The drawing under review shows one solid part. Ordinate dimensions are in mm from its lowest x, y, z. Coordinates: 2 decimals unless noted, no trailing zeros. Order: outer loops, then holes, each group sorted by start corner. A loop starts at its lowest first (then second) coordinate and runs counter-clockwise, first axis right, second up. Notation, with made-up numbers: (14, -38) -> (43, -38) arc R20 cw to (43, -26) -> close; hole circle Ø7 at (-34.75, 18). An arc over 180 degrees is marked (long way). Use a Markdown table: item, result. Add a question column.
Q1. Add section B-B (y = 71). State the section outline as (x, z) points, then the cut area to 3 significant figures.
Q2. Insertion check: pin 1 (2.5 mm diameter, centred on y = 71, z = 16, fed in from -X). The pin has a flat end and moves straight along its axis. Give the tip position at first contact, or say it passes through.
Q3. Wall thickness on probe 1 along Z at (x, y) = (0.85, 14); probe 2 along Y at (x, z) = (2.7, 15): over which ranges is each line inside the solid? List them lowest first.
Q4. Add section A-A (z = 16). State the section outline as (x, y) points.
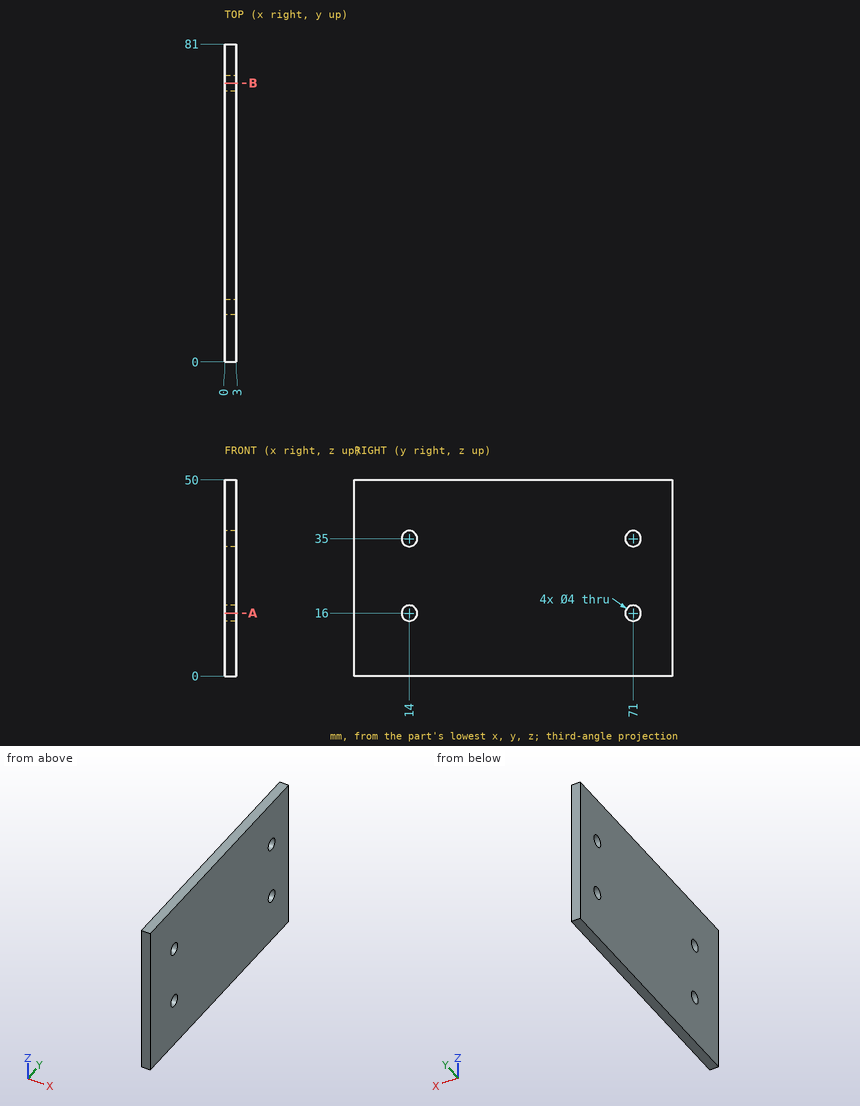
Established:
| question | item | result |
|---|---|---|
| 1 | outline | (0, 0) -> (3, 0) -> (3, 14) -> (0, 14) -> close; (0, 18) -> (3, 18) -> (3, 33) -> (0, 33) -> close; (0, 37) -> (3, 37) -> (3, 50) -> (0, 50) -> close |
| 1 | area | 126 mm^2 |
| 2 | pin 1 | through |
| 3 | probe 1 | 0 to 14, 18 to 33, 37 to 50 |
| 3 | probe 2 | 0 to 12.27, 15.73 to 69.27, 72.73 to 81 |
| 4 | outline | (0, 0) -> (3, 0) -> (3, 12) -> (0, 12) -> close; (0, 16) -> (3, 16) -> (3, 69) -> (0, 69) -> close; (0, 73) -> (3, 73) -> (3, 81) -> (0, 81) -> close |
